Could you check a few things on this drawing? It's one solid part, dimensions in mm from its lowest x, y, z. Round coordinates to 2 decimals unless told otherwise and drop trailing zeros. Write each loop counter-clockwise with the first axis right and the second up, starting at its lowest first coordinate (ties: lowest second). Pieces come first, ordered by that corner, then holes. Notation, with made-up numbers: (-33.75, 60.5) -> (12.25, 60.5) arc R14 ccw to (12.25, 82.5) -> close; hole circle Ø9 at (32.5, 87). An arc over 180 degrees is marked (long way). Return JSON: item names as keys, results as strings.
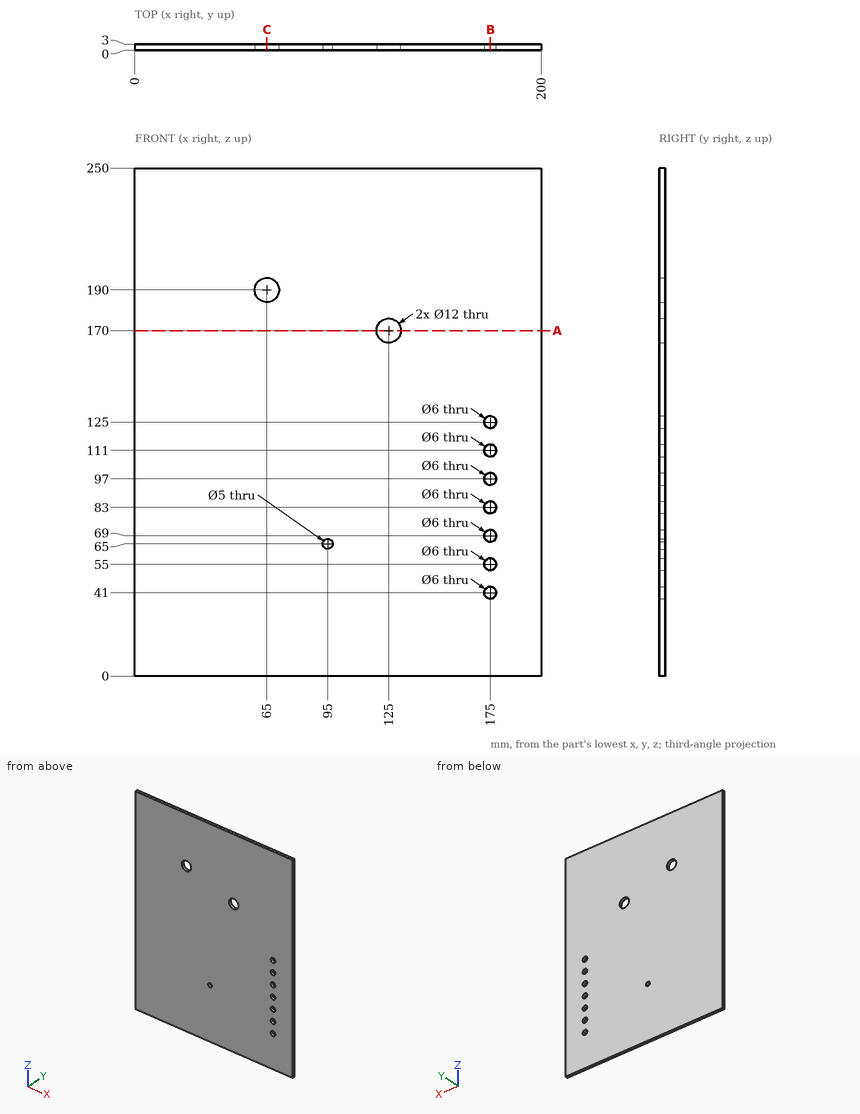
1) I want a section at B-B, the plane x = 175. Count the separate pieces of the cut face and the enclosed holes in it, and give its area (3 significant figures).
Return value:
{"separate pieces": "8", "enclosed holes": "0", "area": "624 mm²"}
2) I want a section at A-A, the plane z = 170. Please give me the cut outline in (x, y), and give its area (3 significant figures).
Return value:
{"outline": "(0, 0) -> (119, 0) -> (119, 3) -> (0, 3) -> close; (131, 0) -> (200, 0) -> (200, 3) -> (131, 3) -> close", "area": "564 mm²"}
3) Will this pin go through, and if not, where does the flat tip stop? pin 1 Ø5 at (x, z) = (175, 83) entering from +Y.
Return value:
{"pin 1": "through"}
4) I want a section at C-C, the plane x = 65. Please give me the cut outline in (y, z), and give its area (3 significant figures).
Return value:
{"outline": "(0, 0) -> (3, 0) -> (3, 184) -> (0, 184) -> close; (0, 196) -> (3, 196) -> (3, 250) -> (0, 250) -> close", "area": "714 mm²"}
5) If I drill on probe 1 along X at (y, z) = (1.3, 83); probe 2 along Z at (x, y) = (95, 1.4); probe 3 along X at (y, z) = (2.95, 173), over which ranges is the centre line in solid material (lowest first)? Write a range as [from, to].
Return value:
{"probe 1": "[0, 172], [178, 200]", "probe 2": "[0, 62.5], [67.5, 250]", "probe 3": "[0, 119.8], [130.2, 200]"}
